Study the drawing (mm; zero at the part's minimum x, y, z) and answer. A direction names the side the tool comes from. Coordinates: 2 decimals unless noted, no trailing zeros. Write each loop counter-clockwise with the first axis right and the second up, starting at its lowest first coordinate (ties: lowest second). Pieces come first, ordered by that corner, then holes. Notation, with made-up numbers: M 50,-21.75 L 84,-21.75 A16 cw 84,-15.75 Z; hole C 67.5,32.5 d3. An arc over 180 degrees is marked long. Answer as CSV lines item,"result". Start each with the question number.
(1) A cutting plane is placed at A-A on z = 7. Give the vertices of the cut face in (x, y) (3 decimals), then the cut area to 3 significant figures.
(2) A cutting plane is placed at B-B on x = 4.75. Give the vertices of the cut face in (y, z), then the cut area to 4 significant figures.
(3) The mould has two halves that part along X. Classify the marked faces 4, 5, 6 and 7: released by +X, released by -X, zero draft, split by the parting line, or undercut.
(4) A cutting plane is placed at C-C on y = 20. Give the vertices of the cut face in (x, z) (3 decimals), then the cut area to 3 significant figures.
(5) Find the intervals of material crossed by L1, parallel to X at y = 4.25, z = 7; L2, parallel to X at y = 20, z = 4.75 (3 decimals); L3, parallel to Y at x = 31, z = 5.25, in increasing order. Write a range as [from, to].
(6) Flat-ended cylindrical pins translate along their axes: P1, Ø3, axis at x = 36, z = 1.5, coming from the +Y side; P2, Ø1, axis at x = 32, y = 30, coming from the -Z side; P3, Ø2, axis at y = 10.5, z = 9, coming from the -X side (3 decimals); P4, Ø4, axis at y = 23.5, z = 9.5, coming from the +X side (3 decimals). Find the tip coordinate at first contact, or state that the pin passes through.
(7) A cutting plane is placed at D-D on z = 1.25. Give the vertices of the cut face in (x, y) (3 decimals), then the cut area to 3 significant figures.
(8) For the marked faces 1, 2 and 3, determine the directions among +Z, -Z, +X, -X, +Y, -Y from which every point of the face is accessible in a straight line to the end or side of a thin tool.
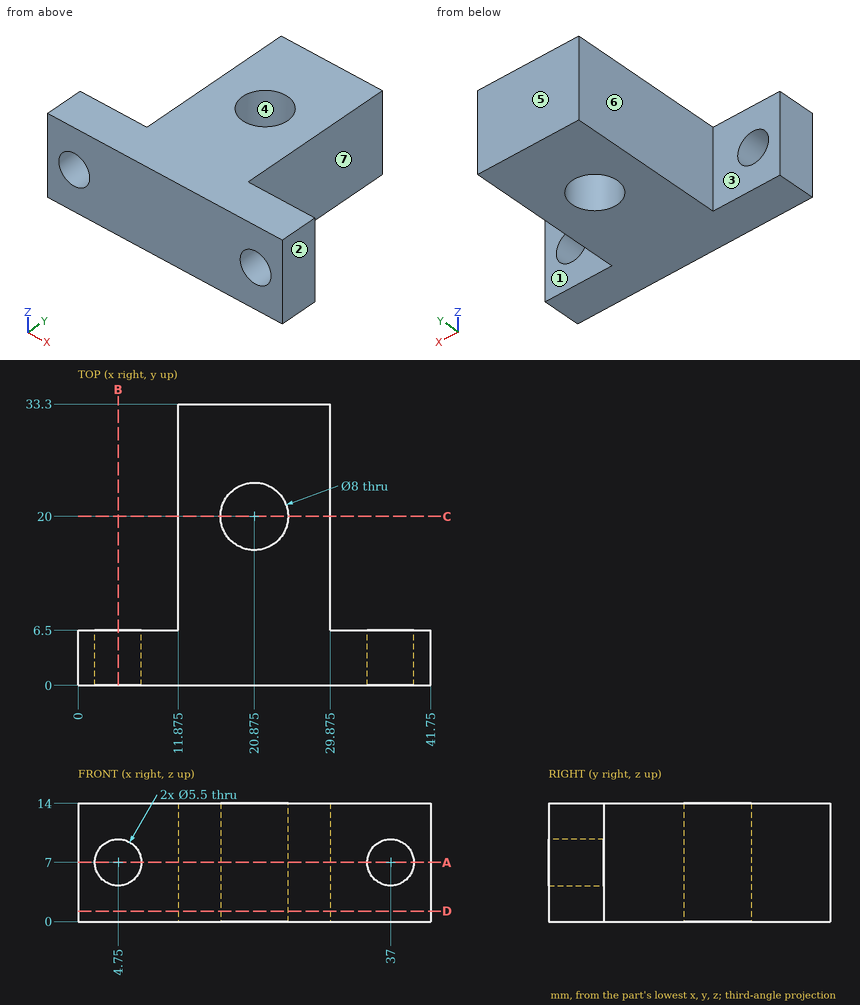
Here are the results:
1,outline,"M 0,0 L 2,0 L 2,6.5 L 0,6.5 Z; M 7.5,0 L 34.25,0 L 34.25,6.5 L 29.875,6.5 L 29.875,33.3 L 11.875,33.3 L 11.875,6.5 L 7.5,6.5 Z; M 39.75,0 L 41.75,0 L 41.75,6.5 L 39.75,6.5 Z; hole C 20.875,20 d8"
1,area,"632 mm^2"
2,outline,"M 0,0 L 6.5,0 L 6.5,4.25 L 0,4.25 Z; M 0,9.75 L 6.5,9.75 L 6.5,14 L 0,14 Z"
2,area,"55.25 mm^2"
3,face 4,"undercut"
3,face 5,"zero draft"
3,face 6,"released by -X"
3,face 7,"released by +X"
4,outline,"M 11.875,0 L 16.875,0 L 16.875,14 L 11.875,14 Z; M 24.875,0 L 29.875,0 L 29.875,14 L 24.875,14 Z"
4,area,"140 mm^2"
5,L1,"x = [0, 2], [7.5, 34.25], [39.75, 41.75]"
5,L2,"x = [11.875, 16.875], [24.875, 29.875]"
5,L3,"y = [0, 6.5]"
6,P1,"stops at y = 6.5"
6,P2,"passes through"
6,P3,"stops at x = 11.875"
6,P4,"stops at x = 29.875"
7,outline,"M 0,0 L 41.75,0 L 41.75,6.5 L 29.875,6.5 L 29.875,33.3 L 11.875,33.3 L 11.875,6.5 L 0,6.5 Z; hole C 20.875,20 d8"
7,area,"704 mm^2"
8,face 1,"+Z, -Z, +X, +Y"
8,face 2,"+Z, -Z, +X, +Y, -Y"
8,face 3,"+Z, -Z, -X, +Y"
